from build123d import *

# Parameters (mm, degrees)
SKETCH_1_W               = 186
SKETCH_1_H               = 110
EXTRUDE_1_DEPTH          = 1
SKETCH_2_R               = 1.6
CUT_EXTRUDE_1_DEPTH      = 2
EXTRUDE_2_DEPTH          = 1
SKETCH_6_R               = 120
CUT_EXTRUDE_2_DEPTH      = 2
SKETCH_8_W               = 186
SKETCH_8_H               = 2
EXTRUDE_3_DEPTH          = 1
SKETCH_7_R               = 1.25
SKETCH_7_R_2             = 1.6
CUT_EXTRUDE_3_DEPTH      = 2
CUT_EXTRUDE_4_DEPTH      = 2
SKETCH_10_W              = 8
SKETCH_10_H              = 15
CUT_EXTRUDE_5_DEPTH      = 2
SKETCH_11_W              = 150
SKETCH_11_H              = 47.5
CUT_EXTRUDE_6_DEPTH      = 2
CHAMFER_2_SIZE           = 5
SKETCH_12_R              = 1.6
CUT_EXTRUDE_7_DEPTH      = 2
SKETCH_14_W              = 3
SKETCH_14_H              = 36.77
CUT_EXTRUDE_8_DEPTH      = 1
CUT_EXTRUDE_8_DEPTH_BACK = 2
SKETCH_15_W              = 5
SKETCH_15_H              = 36.77
EXTRUDE_4_DEPTH          = 1
SKETCH_16_W              = 6
SKETCH_16_H              = 15
CUT_EXTRUDE_9_DEPTH      = 2
CHAMFER_1_SIZE           = 3
FILLET_1_R               = 2


with BuildPart() as part:
    # 草图1 → 凸台-拉伸1 (new body)
    with BuildSketch(Plane(origin=(0, 0, 0), x_dir=(1, 0, 0), z_dir=(0, 1, 0))):
        Rectangle(SKETCH_1_W, SKETCH_1_H)
    extrude(amount=EXTRUDE_1_DEPTH)

    # 草图2 → 切除-拉伸1 (cut, through all)
    with BuildSketch(Plane(origin=(0, 1, 0), x_dir=(1, 0, 0), z_dir=(0, 1, 0))):
        with Locations((90, 15.38)):
            Circle(SKETCH_2_R)
        with Locations((90, 35.38)):
            Circle(SKETCH_2_R)
        with Locations((-90, 35.38)):
            Circle(SKETCH_2_R)
        with Locations((-90, 15.38)):
            Circle(SKETCH_2_R)
    extrude(amount=-CUT_EXTRUDE_1_DEPTH, mode=Mode.SUBTRACT)

    # 草图5 → 凸台-拉伸2 (add)
    with BuildSketch(Plane(origin=(0, 1, 0), x_dir=(1, 0, 0), z_dir=(0, 1, 0))):
        Polygon((-108, -86), (108, -86), (108, -36), (93, -36), (93, -55), (-93, -55), (-93, -36), (-108, -36), align=None)
    extrude(amount=-EXTRUDE_2_DEPTH)

    # 草图6 → 切除-拉伸2 (cut, through all)
    with BuildSketch(Plane(origin=(0, 1, 0), x_dir=(1, 0, 0), z_dir=(0, 1, 0))):
        with Locations((0, -155.12)):
            Circle(SKETCH_6_R)
    extrude(amount=-CUT_EXTRUDE_2_DEPTH, mode=Mode.SUBTRACT)

    # 草图8 → 凸台-拉伸3 (add)
    with BuildSketch(Plane(origin=(0, 1, 0), x_dir=(1, 0, 0), z_dir=(0, 1, 0))):
        with Locations((0, 56)):
            Rectangle(SKETCH_8_W, SKETCH_8_H)
    extrude(amount=-EXTRUDE_3_DEPTH)

    # 草图7 → 切除-拉伸3 (cut, through all)
    with BuildSketch(Plane(origin=(0, 1, 0), x_dir=(1, 0, 0), z_dir=(0, 1, 0))):
        with Locations((47.5, 46.38)):
            Circle(SKETCH_7_R)
        with Locations((47.5, 53.88)):
            Circle(SKETCH_7_R)
        with Locations((102, -74.62)):
            Circle(SKETCH_7_R_2)
        with Locations((102, -54.62)):
            Circle(SKETCH_7_R_2)
        with Locations((-102, -54.62)):
            Circle(SKETCH_7_R_2)
        with Locations((-102, -74.62)):
            Circle(SKETCH_7_R_2)
        with Locations((-47.5, 53.88)):
            Circle(SKETCH_7_R)
        with Locations((-47.5, 46.38)):
            Circle(SKETCH_7_R)
    extrude(amount=-CUT_EXTRUDE_3_DEPTH, mode=Mode.SUBTRACT)

    # 草图9 → 切除-拉伸4 (cut, through all)
    with BuildSketch(Plane(origin=(0, 1, 0), x_dir=(1, 0, 0), z_dir=(0, 1, 0))):
        with BuildLine():
            Line((55, 52.23), (55, 20.23))
            Line((55, 20.23), (40, 20.23))
            Line((40, 20.23), (40, 52.23))
            Line((40, 52.23), (40, 66.764572681))
            ThreePointArc((40, 66.764572681), (40.878679656, 68.885893025), (43, 69.764572681))
            Line((43, 69.764572681), (52, 69.764572681))
            ThreePointArc((52, 69.764572681), (54.121320344, 68.885893025), (55, 66.764572681))
            Line((55, 66.764572681), (55, 52.23))
        make_face()
        with BuildLine():
            Line((-40, 66.764572681), (-40, 52.23))
            Line((-40, 52.23), (-40, 20.23))
            Line((-40, 20.23), (-55, 20.23))
            Line((-55, 20.23), (-55, 52.23))
            Line((-55, 52.23), (-55, 66.764572681))
            ThreePointArc((-55, 66.764572681), (-54.121320344, 68.885893025), (-52, 69.764572681))
            Line((-52, 69.764572681), (-43, 69.764572681))
            ThreePointArc((-43, 69.764572681), (-40.878679656, 68.885893025), (-40, 66.764572681))
        make_face()
    extrude(amount=-CUT_EXTRUDE_4_DEPTH, mode=Mode.SUBTRACT)

    # 草图10 → 切除-拉伸5 (cut, through all)
    with BuildSketch(Plane(origin=(0, 1, 0), x_dir=(1, 0, 0), z_dir=(0, 1, 0))):
        with Locations((-36, 27.73)):
            Rectangle(SKETCH_10_W, SKETCH_10_H)
    extrude(amount=-CUT_EXTRUDE_5_DEPTH, mode=Mode.SUBTRACT)

    # 草图11 → 切除-拉伸6 (cut, through all)
    with BuildSketch(Plane(origin=(0, 1, 0), x_dir=(1, 0, 0), z_dir=(0, 1, 0))):
        with Locations((0, -7.52)):
            Rectangle(SKETCH_11_W, SKETCH_11_H)
    extrude(amount=-CUT_EXTRUDE_6_DEPTH, mode=Mode.SUBTRACT)

    # 倒角2
    chamfer_2_edges = [part.edges().sort_by_distance(p)[0] for p in [
        (75, 0.5, -16.23),
        (75, 0.5, 31.27),
        (-75, 0.5, 31.27),
        (-75, 0.5, -16.23),
    ]]
    chamfer(chamfer_2_edges, length=CHAMFER_2_SIZE)

    # 草图12 → 切除-拉伸7 (cut, through all)
    with BuildSketch(Plane(origin=(0, 1, 0), x_dir=(1, 0, 0), z_dir=(0, 1, 0))):
        with Locations((-87, -0.52)):
            Circle(SKETCH_12_R)
        with Locations((-87, -14.52)):
            Circle(SKETCH_12_R)
        with Locations((87, -14.52)):
            Circle(SKETCH_12_R)
        with Locations((87, -0.52)):
            Circle(SKETCH_12_R)
    extrude(amount=-CUT_EXTRUDE_7_DEPTH, mode=Mode.SUBTRACT)

    # 草图14 → 切除-拉伸8 (cut, two sides)
    with BuildSketch(Plane(origin=(0, 1, 0), x_dir=(1, 0, 0), z_dir=(0, 1, 0))) as cut_extrude_8_sk:
        with Locations((-56.5, 38.615)):
            Rectangle(SKETCH_14_W, SKETCH_14_H)
        with Locations((56.5, 38.615)):
            Rectangle(SKETCH_14_W, SKETCH_14_H)
    extrude(amount=CUT_EXTRUDE_8_DEPTH, mode=Mode.SUBTRACT)
    extrude(cut_extrude_8_sk.sketch, amount=-CUT_EXTRUDE_8_DEPTH_BACK, mode=Mode.SUBTRACT)

    # 草图15 → 凸台-拉伸4 (add)
    with BuildSketch(Plane(origin=(0, 1, 0), x_dir=(1, 0, 0), z_dir=(0, 1, 0))):
        with Locations((42.5, 38.615)):
            Rectangle(SKETCH_15_W, SKETCH_15_H)
        with Locations((-42.5, 38.615)):
            Rectangle(SKETCH_15_W, SKETCH_15_H)
    extrude(amount=-EXTRUDE_4_DEPTH)

    # 草图16 → 切除-拉伸9 (cut, through all)
    with BuildSketch(Plane(origin=(0, 1, 0), x_dir=(1, 0, 0), z_dir=(0, 1, 0))):
        with Locations((-42, 27.73)):
            Rectangle(SKETCH_16_W, SKETCH_16_H)
    extrude(amount=-CUT_EXTRUDE_9_DEPTH, mode=Mode.SUBTRACT)

    # 倒角1
    chamfer_1_edges = [part.edges().sort_by_distance(p)[0] for p in [
        (-58, 0.5, -57),
        (58, 0.5, -57),
        (-45, 0.5, -57),
        (45, 0.5, -57),
        (-93, 0.5, 36),
        (93, 0.5, 36),
        (108, 0.5, 36),
        (108, 0.5, 86),
        (-108, 0.5, 86),
        (-108, 0.5, 36),
        (93, 0.5, -57),
        (-93, 0.5, -57),
    ]]
    chamfer(chamfer_1_edges, length=CHAMFER_1_SIZE)

    # 圆角1
    fillet_1_edges = [part.edges().sort_by_distance(p)[0] for p in [
        (-32, 0.5, -35.23),
        (-32, 0.5, -20.23),
        (-58, 0.5, -20.23),
        (58, 0.5, -20.23),
        (45, 0.5, -20.23),
        (-45, 0.5, -35.23),
        (-98.093963117, 0.5, 86),
        (98.093963117, 0.5, 86),
    ]]
    fillet(fillet_1_edges, radius=FILLET_1_R)


solid = part.part
Work out the finished part from the listing and answer in its coordinate system (mm). A direction names the side the tool comes from. Round coordinates to 2 decimals unless told otherwise and drop trailing zeros. Write each loop counter-clockwise with the first axis right and the second up, starting at its lowest first coordinate (ties: lowest second). Pieces come first, ordered by that corner, then holes.
1) A cutting plane is placed at C-C (y = 0.55). Give the number of separate pieces and of enclosed holes in the cut face, plus the area to 3 significant figures.
2) The mould has two halves that part along Z. Classify faces 3 (the cylindrical face through (1.59, 0.51, 35.13)), 4 (the flat face through (-1, 0, -23)), 5 (the flat face through (-72.535, 0.507, 28.735)): pulls with the +Z half, pulls with the -Z half, needs draft (parallel to the pull), parting line crosses it, or undercut.
3) A cutting plane is placed at B-B (x = -12). Give the vertices of the cut face in (y, z).
4) A cutting plane is placed at D-D (z = -29). Give the vertices of the cut face in (x, y).
5) Given pin 1 Ø2.5 at (x, z) = (87, 0.52) entering from -Y; pin 2 Ø0.5 at (y, z) = (0.5, -29) entering from -X, each flat-ended and moving along its own axis, determine where each tip first touches the part or whether it passes through.
6) A tool of negligible diameter and unlimited length cuts with its end or side. For faces 1 (the flat face through (-1, 1, -23)), 2 (the flat face through (72.535, 0.507, 28.735)), from which of +Z, -Z, +X, -X, +Y, -Y can it reach the whole face along a straight path? Write none if from no direction.
7) A cutting plane is placed at A-A (z = -47). Give the vertices of the cut face in (x, y).
8) Straight lines are drawn through the part: line 1 (Z direction, x = -102, y = 0.3); line 2 (X direction, y = 0.25, z = -51); line 3 (X direction, y = 0.5, z = -29). For each, find the intervals that lie inside material, in ascending order.
Completed:
1. separate pieces: 1
1. enclosed holes: 13
1. area: 12,700 mm2
2. face 3: pulls with the +Z half
2. face 4: needs draft
2. face 5: undercut
3. outline: (0, -57) - (1, -57) - (1, -16.23) - (0, -16.23) - close; (0, 31.27) - (1, 31.27) - (1, 35.72) - (0, 35.72) - close
4. outline: (-93, 0) - (-58, 0) - (-58, 1) - (-93, 1) - close; (-32, 0) - (45, 0) - (45, 1) - (-32, 1) - close; (58, 0) - (93, 0) - (93, 1) - (58, 1) - close
5. pin 1: passes through
5. pin 2: stops at x = -93
6. face 1: +Z, -Z, +X, -X, +Y
6. face 2: +Y, -Y
7. outline: (-93, 0) - (-58, 0) - (-58, 1) - (-93, 1) - close; (-45, 0) - (45, 0) - (45, 1) - (-45, 1) - close; (58, 0) - (93, 0) - (93, 1) - (58, 1) - close
8. line 1: z = 36 to 53.02, 56.22 to 73.02, 76.22 to 86
8. line 2: x = -93 to -58, -45 to 45, 58 to 93
8. line 3: x = -93 to -58, -32 to 45, 58 to 93
